```python
from build123d import *

# Parameters (mm, degrees)
F0_R     = 35
F0_W     = 4
F0_H     = 2
F0_W_2   = 2
F0_H_2   = 13
F0_H_3   = 10
F1_DEPTH = 5


with BuildPart() as f1:
    # F0 (on Top) → F1 (new body)
    with BuildSketch(Plane.XY):
        with Locations((-33.946003, 33.575995)):
            Circle(F0_R)
        Polygon((-54.261632, 19.790954), (-48.261632, 19.790954), (-48.261632, 17.790954), (-50.261632, 17.790954), (-48.261632, 12.791132), (-50.261632, 11.791284), (-51.262511, 14.790954), (-52.261632, 11.790954), (-54.261632, 12.791132), (-52.261632, 17.790954), (-54.261632, 17.790954), align=None, mode=Mode.SUBTRACT)
        Polygon((-45.261632, 21.791132), (-43.261632, 21.791132), (-43.261632, 9.791132), (-45.261632, 9.791132), (-45.261632, 14.791132), (-47.261632, 14.791132), (-47.261632, 16.791132), (-45.261632, 16.791132), align=None, mode=Mode.SUBTRACT)
        Polygon((-41.261632, 21.791132), (-40.235692, 21.791132), (-40.235692, 9.791132), (-42.235692, 9.791132), (-42.235692, 21.791132), align=None, mode=Mode.SUBTRACT)
        Polygon((-39.235692, 14.791132), (-39.235692, 16.791132), (-37.235692, 19.791132), (-36.235692, 19.791132), (-36.235692, 16.791132), (-37.235692, 16.791132), (-37.235692, 14.791132), (-36.235692, 14.791132), (-36.235692, 11.791132), (-37.235692, 11.791132), align=None, mode=Mode.SUBTRACT)
        Polygon((-35.235692, 11.791132), (-35.235692, 19.791132), (-33.235692, 16.791132), (-33.235692, 14.791132), align=None, mode=Mode.SUBTRACT)
        Polygon((-32.235692, 21.791132), (-30.235692, 21.791132), (-30.235692, 9.791132), (-32.235692, 9.791132), (-32.235692, 11.791132), (-32.235692, 19.791132), align=None, mode=Mode.SUBTRACT)
        Polygon((-27.235692, 4.777636), (-27.235692, 10.777636), (-26.235692, 10.777636), (-25.235692, 10.777636), (-25.235692, 9.777636), (-23.235692, 9.777636), (-23.235692, 7.777636), (-25.235692, 7.777636), (-25.235692, 6.777636), (-21.235692, 6.777636), (-21.235692, 10.777636), (-20.235692, 10.777636), (-19.235692, 10.777636), (-19.235692, 4.777636), align=None, mode=Mode.SUBTRACT)
        Polygon((-18.235692, 11.777636), (-28.235692, 11.777636), (-28.235692, 13.777636), (-24.235692, 13.777636), (-24.235692, 15.777636), (-22.235692, 15.777636), (-22.235692, 13.777636), (-18.235692, 13.777636), align=None, mode=Mode.SUBTRACT)
        Polygon((-23.235692, 16.791132), (-24.235692, 16.791132), (-26.235692, 17.79098), (-26.235692, 18.791284), (-24.235692, 19.791132), (-23.235692, 19.791132), (-23.235692, 18.791132), (-24.235692, 18.791132), (-24.235692, 17.79098), (-23.235692, 17.79098), align=None, mode=Mode.SUBTRACT)
        Polygon((-22.235692, 19.791132), (-20.235692, 18.79098), (-20.235692, 17.79098), (-22.235692, 16.791132), align=None, mode=Mode.SUBTRACT)
        Polygon((-28.235692, 22.791132), (-18.235692, 22.791132), (-18.235692, 20.791132), (-28.235692, 20.791132), (-28.235692, 21.791132), align=None, mode=Mode.SUBTRACT)
        with Locations((-23.235692, 24.777636)):
            Rectangle(F0_W, F0_H, mode=Mode.SUBTRACT)
        Polygon((-48.946003, 52.576141), (-48.946003, 54.576141), (-38.946003, 54.576141), (-38.946003, 52.576141), (-42.945711, 52.576141), (-38.946003, 44.575995), (-40.946039, 43.576068), (-43.946094, 49.575812), (-46.946003, 43.575995), (-48.945828, 44.575907), (-44.945711, 52.576141), align=None, mode=Mode.SUBTRACT)
        with Locations((-35.946003, 49.075995)):
            Rectangle(F0_W_2, F0_H_2, mode=Mode.SUBTRACT)
        Polygon((-30.946003, 40.575995), (-30.946003, 46.575995), (-28.946003, 46.575995), (-28.946003, 42.575995), (-19.946003, 42.575995), (-19.946003, 40.575995), (-28.946003, 40.575995), align=None, mode=Mode.SUBTRACT)
        Polygon((-22.946003, 48.575995), (-30.946003, 48.575995), (-28.959546, 50.575995), (-24.959546, 50.575995), align=None, mode=Mode.SUBTRACT)
        Polygon((-31.946003, 49.575995), (-31.946003, 57.575995), (-29.959546, 55.579393), (-29.959546, 51.575995), align=None, mode=Mode.SUBTRACT)
        Polygon((-28.959546, 56.575995), (-30.946003, 58.575995), (-22.946003, 58.575995), (-24.959546, 56.575995), align=None, mode=Mode.SUBTRACT)
        Polygon((-23.959546, 55.575995), (-21.946003, 57.575995), (-21.946003, 49.575995), (-23.959546, 51.575995), align=None, mode=Mode.SUBTRACT)
        with Locations((-20.235692, 53.575995)):
            Rectangle(F0_W_2, F0_H_3, mode=Mode.SUBTRACT)
    extrude(amount=F1_DEPTH)


solid = f1.part
```
Here's how the part is built. I have some questions about the finished solid (model axes, mm). Coordinates: 2 decimals unless noted, no trailing zeros. Write each loop counter-clockwise with the first axis right and the second up, starting at its lowest first coordinate (ties: lowest second). Pieces come first, ordered by that corner, then holes. Notation, with made-up numbers: (8, -32) -> (66, -32) arc R26 ccw to (66, -18) -> close; hole circle Ø6 at (77.25, -25.5). An arc over 180 degrees is marked (long way). Use a Markdown table: item, result. Add a question column.
(1) I'm going to push flat-ended pins straight in: P1, Ø1.6, axis at y = 21.5, z = 3.5, coming from the +X side; P2, Ø0.6, axis at y = 22, z = 2.5, coming from the -X side; P3, Ø0.6, axis at y = 12.5, z = 2.5, coming from the -X side; P4, Ø12, axis at x = -36, y = 24, coming from the -Z side. Where does each tip first touch, or does it pass through?
(2) If we section it at C-C, the plane z = 3.05: State how many separate pieces and enclosed holes the cut face has, and give its area (3 significant figures).
(3) If we section it at B-B, the plane x = -8.5: Write out the boundary of the cut face in (y, z), and give its area (3 significant figures).
(4) Please list where these lines run through material, in increasing order: line 1 (Y direction, x = -44, z = 0.5); line 2 (X direction, y = 43, z = 4.75); line 3 (X direction, y = 20, z = 4.65).
(5) If we section it at A-A, the plane y = 61: Write out the boundary of the cut face in (x, z).
Outcome:
| question | item | result |
|---|---|---|
| 1 | P1 | stops at x = -0.81 |
| 1 | P2 | stops at x = -67.08 |
| 1 | P3 | stops at x = -62.11 |
| 1 | P4 | stops at z = 0 |
| 2 | separate pieces | 1 |
| 2 | enclosed holes | 20 |
| 2 | area | 3,430 mm^2 |
| 3 | outline | (9.54, 0) -> (57.61, 0) -> (57.61, 5) -> (9.54, 5) -> close |
| 3 | area | 240 mm^2 |
| 4 | line 1 | y = 0.05 to 9.79, 21.79 to 49.47, 54.58 to 67.1 |
| 4 | line 2 | x = -67.65 to -36.95, -34.95 to -30.95, -28.95 to -0.24 |
| 4 | line 3 | x = -66.21 to -45.26, -43.26 to -42.24, -40.24 to -32.24, -30.24 to -1.69 |
| 5 | outline | (-55.69, 0) -> (-12.2, 0) -> (-12.2, 5) -> (-55.69, 5) -> close |
